```python
from build123d import *

# Parameters (mm, degrees)
F0_R           = 4
F1_DEPTH       = 486
F4_D           = 5
F4_DEPTH       = 20
F4_TIP         = 1.5021515476
F4_ON_F2_D     = 5
F4_ON_F2_DEPTH = 20
F4_ON_F2_TIP   = 1.5021515476
F5_SIZE        = 0.5


with BuildPart() as f1:
    # F0 (on Right) → F1 (new body)
    with BuildSketch(Plane.YZ):
        Circle(F0_R)
    extrude(amount=F1_DEPTH)

    # F4
    with Locations(Plane(origin=(0, 0, 0), x_dir=(0, -1, 0), z_dir=(-1, 0, 0))):
        with Locations((0, 0)):
            Hole(F4_D / 2, depth=F4_DEPTH)
            with Locations((0, 0, -(F4_DEPTH + F4_TIP / 2))):  # 118° drill point
                Cone(0, F4_D / 2, F4_TIP, mode=Mode.SUBTRACT)

    # F4 on F2
    with Locations(Plane.YZ.offset(486)):
        with Locations((0, 0)):
            Hole(F4_ON_F2_D / 2, depth=F4_ON_F2_DEPTH)
            with Locations((0, 0, -(F4_ON_F2_DEPTH + F4_ON_F2_TIP / 2))):  # 118° drill point
                Cone(0, F4_ON_F2_D / 2, F4_ON_F2_TIP, mode=Mode.SUBTRACT)

    # F5
    f5_edges = [f1.edges().sort_by_distance(p)[0] for p in [
        (486, -4, 0),
        (0, -4, 0),
    ]]
    chamfer(f5_edges, length=F5_SIZE)


solid = f1.part
```
Read the model definition and answer for the solid it produces. Units are mm, in the model's axes. Give positions to 0.01 mm unless a question says otherwise; leave off trailing zeros. Loops run counter-clockwise (first coordinate to the right, second up) from the corner with the lowest first, then second, coordinate; pieces in that order, holes last.
Item 1: Each of these flat-tipped pins is pushed along its axis until it touches: pin 1 Ø4.5 at (y, z) = (0, 0) entering from +X; pin 2 Ø1.5 at (x, z) = (176, -2.5) entering from -Y; pin 3 Ø3 at (x, y) = (400, -2.5) entering from -Z. Where does it stop, or does it pass through?
Item 2: Find the intervals of material crossed by line 1 along Z through (x, y) = (5.5, 0); line 2 along X through (y, z) = (3.25, -2.25); line 3 along Y through (x, z) = (222.5, -2.5), in increasing order.
Item 3: The part is cut by section A-A (x = 154.5). Write down the section's boundary in (y, z), and give its area (3 significant figures).
Taken from the geometry:
1. pin 1: stops at x = 465.85
1. pin 2: stops at y = -3.6
1. pin 3: stops at z = -3.87
2. line 1: z = -4 to -2.5, 2.5 to 4
2. line 2: x = 0.45 to 485.55
2. line 3: y = -3.12 to 3.12
3. outline: circle Ø8 at (0, 0)
3. area: 50.3 mm2
